Read the model definition and answer for the solid it produces. Units are mm, in the model's axes. Face numbers are marked on the shaded views. A direction names the side the tool comes from. Coordinates: 2 decimals unless noted, no trailing zeros. Write each loop counter-clockwise with the first axis right and the second up, starting at its lowest first coordinate (ties: lowest second). Pieces come first, ordered by that corner, then holes.
(1) Given pin 1 (4 mm diameter, centred on y = 2.5, z = 81, fed in from -X); pin 2 (2 mm diameter, centred on y = -2.5, z = 71.5, fed in from +X); pin 3 (6 mm diameter, centred on x = 5, z = 11.5, fed in from +Y); pin 4 (2 mm diameter, centred on x = -6.5, z = 52.5, fed in from -Y), each flat-ended and moving along its own axis, determine where each tip first touches the part or whether it passes through.
(2) The part is cut by section B-B, the plane x = -6.5. Determine the outline of the cut face in (y, z).
(3) Which of the six approach directions +Z, -Z, +X, -X, +Y, -Y give full straight-line access (tool end or side, diameter ignored) to the marked faces 1 and 2?
(4) The part is cut by section A-A, the plane z = 77.5. Determine the outline of the cut face in (x, y).
(5) Straight lines are drawn through the part: line 1 along Y through (x, z) = (0, 70.5); line 2 along Z through (x, y) = (4.75, -5.5). For each, find the intervals that lie inside material, in ascending order.
```python
from build123d import *

# Parameters (mm, degrees)
F0_R     = 8.5
F1_DEPTH = 4
F2_R     = 5
F3_DEPTH = 100
F6_R     = 0.5
F7_DEPTH = 169.1


with BuildPart() as f1:
    # F0 (on Top) → F1 (new body)
    with BuildSketch(Plane.XY):
        Circle(F0_R)
    extrude(amount=F1_DEPTH)

    # F2 (on Top) → F3 (join)
    with BuildSketch(Plane.XY):
        Circle(F2_R)
    extrude(amount=F3_DEPTH)

    # F4 (on Right) → F5 (revolve)
    with BuildSketch(Plane.YZ):
        with BuildLine():
            Line((0, 104), (0, 100))
            Line((0, 100), (5, 100))
            ThreePointArc((5, 100), (4.472136, 102.236068), (3, 104))
            Line((3, 104), (0, 104))
        make_face()
        with BuildLine():
            ThreePointArc((0, 105), (1.581139, 104.743416), (3, 104))
            ThreePointArc((3, 104), (2.414214, 105.414214), (1, 106))
            Line((1, 106), (0, 106))
            Line((0, 106), (0, 105))
        make_face()
        with BuildLine():
            Line((0, 105), (0, 104))
            Line((0, 104), (3, 104))
            ThreePointArc((3, 104), (1.581139, 104.743416), (0, 105))
        make_face()
    revolve(axis=Axis((0, 0, 103), (0, 0, -1)))

    # F6 (on face) → F7 (cut)
    with BuildSketch(Plane(origin=(0, 0, 0), x_dir=(1, 0, 0), z_dir=(0, 0, -1))):
        Circle(F6_R)
    extrude(amount=-F7_DEPTH, mode=Mode.SUBTRACT)


solid = f1.part
```
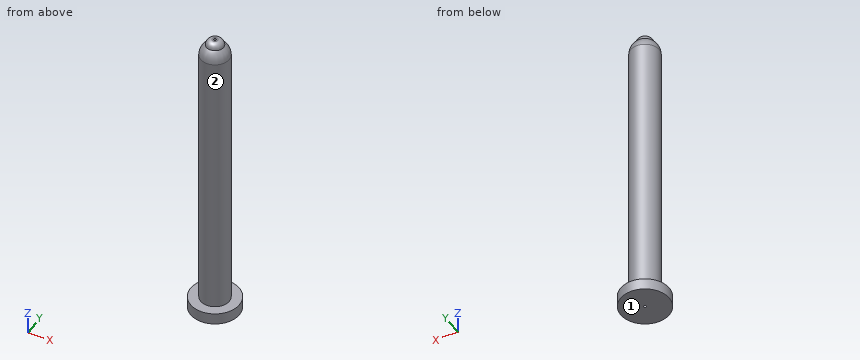
Computed:
1. pin 1: stops at x = -4.97
1. pin 2: stops at x = 4.77
1. pin 3: stops at y = 4.58
1. pin 4: passes through
2. outline: (-5.48, 0) - (5.48, 0) - (5.48, 4) - (-5.48, 4) - close
3. face 1: -Z, +X, -X, +Y, -Y
3. face 2: +Z
4. outline: circle Ø10 at (0, 0); hole circle Ø1 at (0, 0)
5. line 1: y = -5 to -0.5, 0.5 to 5
5. line 2: z = 0 to 4
